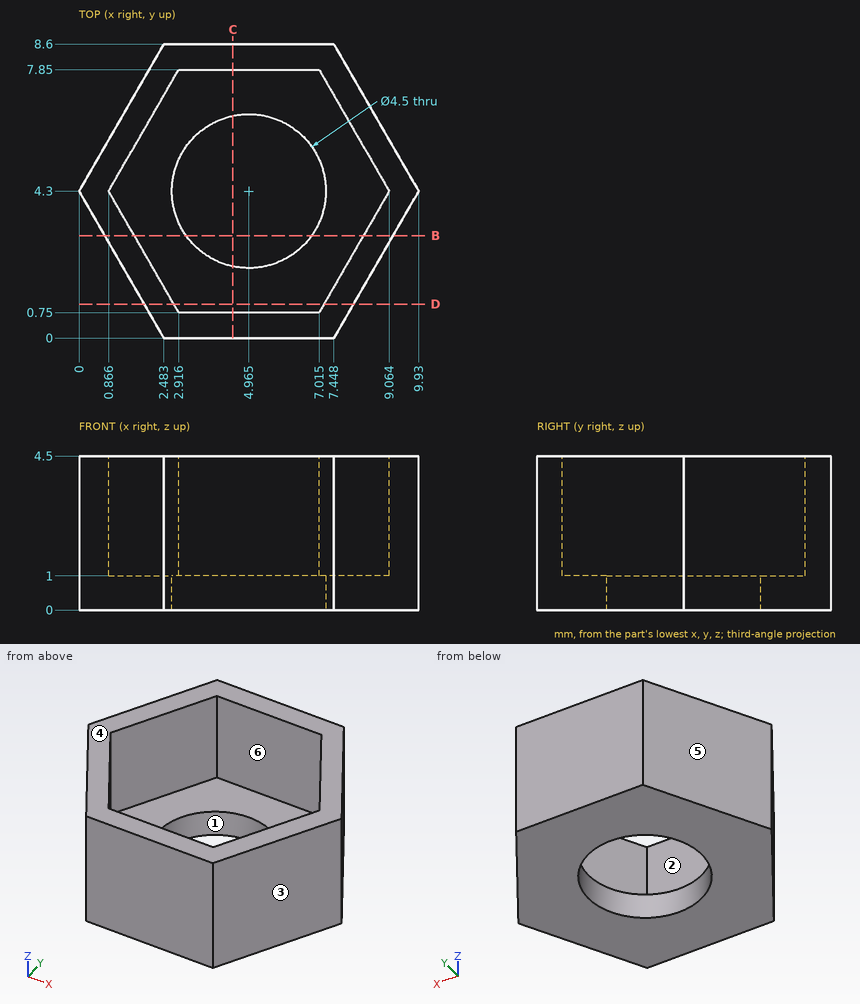
Job drawing, mm, ordinate dimensions from the low corner. One solid piece. A direction names the side the tool comes from. Give positions to 0.01 mm unless a question says otherwise; leave off trailing zeros. Loops run counter-clockwise (first coordinate to the right, second up) from the corner with the lowest first, then second, coordinate; pieces in that order, holes last. Notation, with made-up numbers: M -1,30.25 L 5,30.25 A36 cw 5,68.25 Z; hole C 79,52.5 d2. An arc over 180 degrees is marked long. Answer in a Markdown table with one row per item. Add a question column.
Item 1: Mould opens along X. For the marked faces 3, 4, 5 and 6 say: +X half, -X half, draft (parallel to the pull), parting line (faces both ways), or undercut.
Item 2: Probe probe 1 along Y at (x, z) = (4.5, 2.35); probe 2 along Y at (x, z) = (8.25, 2.05); probe 3 along Z at (x, y) = (8, 3.25). List the from-to ranges inside material, lowest first.
Item 3: Drop flat-ended pins along their axis: P1, Ø2, axis at x = 3, y = 3, coming from the -Z side; P2, Ø2, axis at x = 8.5, z = 2.5, coming from the -Y side; P3, Ø5, axis at x = 4.97, y = 4.3, coming from the +Z side. Give the stop position or say it passes through.
Item 4: Band-saw the part on D-D on y = 1. Give the cut face in (x, z) (1 decimal), then the cut area to 3 significant figures.
Item 5: Band-saw the part on B-B on y = 3. Give the cut face in (x, z).
Item 6: Band-saw the part on C-C on x = 4.5. Give the cut face in (y, z).
Item 7: Tool access for the marked faces 1 and 2: list every direction of +Z, -Z, +X, -X, +Y, -Y with a clear straight run to the whole face (end or side of a thin tool).
Reply:
| question | item | result |
|---|---|---|
| 1 | face 3 | +X half |
| 1 | face 4 | draft |
| 1 | face 5 | -X half |
| 1 | face 6 | undercut |
| 2 | probe 1 | y = 0 to 0.75, 7.85 to 8.6 |
| 2 | probe 2 | y = 1.39 to 2.89, 5.71 to 7.21 |
| 2 | probe 3 | z = 0 to 1 |
| 3 | P1 | stops at z = 0 |
| 3 | P2 | stops at y = 0.09 |
| 3 | P3 | stops at z = 1 |
| 4 | outline | M 1.9,0 L 8,0 L 8,4.5 L 7.2,4.5 L 7.2,1 L 2.8,1 L 2.8,4.5 L 1.9,4.5 Z |
| 4 | area | 12.2 mm^2 |
| 5 | outline | M 0.75,0 L 3.13,0 L 3.13,1 L 1.62,1 L 1.62,4.5 L 0.75,4.5 Z; M 6.8,0 L 9.18,0 L 9.18,4.5 L 8.31,4.5 L 8.31,1 L 6.8,1 Z |
| 6 | outline | M 0,0 L 2.1,0 L 2.1,1 L 0.75,1 L 0.75,4.5 L 0,4.5 Z; M 6.5,0 L 8.6,0 L 8.6,4.5 L 7.85,4.5 L 7.85,1 L 6.5,1 Z |
| 7 | face 1 | +Z, -Z |
| 7 | face 2 | +Z |
